from build123d import *

# Parameters (mm, degrees)
SKETCH2_R           = 41.275
SKETCH2_R_2         = 38.1
SKETCH2_R_3         = 34.925
BOSS_EXTRUDE1_DEPTH = 3.175
SKETCH3_R           = 1.5875
BOSS_EXTRUDE2_DEPTH = 3.175
CUT_EXTRUDE1_DEPTH  = 3.175


with BuildPart() as part:
    # Sketch2 → Boss-Extrude1 (new body)
    with BuildSketch(Plane.XY):
        Circle(SKETCH2_R)
        Circle(SKETCH2_R_2, mode=Mode.SUBTRACT)
        Circle(SKETCH2_R_2)
        Circle(SKETCH2_R_3, mode=Mode.SUBTRACT)
    extrude(amount=BOSS_EXTRUDE1_DEPTH)

    # Sketch3 → Boss-Extrude2 (add)
    with BuildSketch(Plane.XY.offset(3.175)):
        with BuildLine():
            ThreePointArc((-25.891068033, 32.144645295), (-23.333836091, 34.046405365), (-20.6375, 35.745198541))
            Line((-20.6375, 35.745198541), (-26.9875, 46.743721169))
            Line((-26.9875, 46.743721169), (-32.486761314, 43.568721169))
            Line((-32.486761314, 43.568721169), (-26.136761314, 32.570198541))
            Line((-26.136761314, 32.570198541), (-25.891068033, 32.144645295))
        make_face()
        with Locations((-28.149630657, 42.406590512)):
            Circle(SKETCH3_R, mode=Mode.SUBTRACT)
        with BuildLine():
            Line((26.9875, 46.743721169), (20.6375, 35.745198541))
            ThreePointArc((20.6375, 35.745198541), (23.333836091, 34.046405365), (25.891068033, 32.144645295))
            Line((25.891068033, 32.144645295), (26.136761314, 32.570198541))
            Line((26.136761314, 32.570198541), (32.486761314, 43.568721169))
            Line((32.486761314, 43.568721169), (26.9875, 46.743721169))
        make_face()
        with Locations((28.149630657, 42.406590512)):
            Circle(SKETCH3_R, mode=Mode.SUBTRACT)
    extrude(amount=-BOSS_EXTRUDE2_DEPTH)

    # Sketch5 → Cut-Extrude1 (cut)
    with BuildSketch(Plane.XY.offset(3.175)):
        with BuildLine():
            Line((-20.6375, 35.745198541), (0, 0))
            Line((0, 0), (20.6375, 35.745198541))
            ThreePointArc((20.6375, 35.745198541), (0, 41.275), (-20.6375, 35.745198541))
        make_face()
    extrude(amount=-CUT_EXTRUDE1_DEPTH, mode=Mode.SUBTRACT)


solid = part.part
Verification items for the finished model (mm, model axes). A direction names the side the tool comes from. Coordinates: 2 decimals unless noted, no trailing zeros. Write each loop counter-clockwise with the first axis right and the second up, starting at its lowest first coordinate (ties: lowest second). Pieces come first, ordered by that corner, then holes. Notation, with made-up numbers: M 56.25,85.25 L 103.25,85.25 A31 ccw 103.25,113.25 Z; hole C -21,47.25 d4. An arc over 180 degrees is marked long. Use a Markdown table: item, result.
Q1. Sectioned sample at C-C, the plane y = 22. Record the boundary of the cut face in (x, z) (3 decimals).
Reply:
| item | result |
|---|---|
| outline | M -34.923,0 L -27.125,0 L -27.125,3.175 L -34.923,3.175 Z; M 27.125,0 L 34.923,0 L 34.923,3.175 L 27.125,3.175 Z |
Q2. Sectioned sample at D-D, the plane x = 0. Record the boundary of the cut face in (y, z) (3 decimals).
Reply:
| item | result |
|---|---|
| outline | M -41.275,0 L -34.925,0 L -34.925,3.175 L -41.275,3.175 Z |
Q3. Sectioned sample at A-A, the plane y = 0. Record the boundary of the cut face in (x, z) (3 decimals), plus the area to 3 significant figures.
Reply:
| item | result |
|---|---|
| outline | M -41.275,0 L -34.925,0 L -34.925,3.175 L -41.275,3.175 Z; M 34.925,0 L 41.275,0 L 41.275,3.175 L 34.925,3.175 Z |
| area | 40.3 mm² |
Q4. Go/stop test with flat-tipped pins: P1, Ø1.5, axis at x = -2.5, z = 1, coming from the -Y side; P2, Ø1, axis at y = 13, z = 2, coming from the -X side; P3, Ø1, axis at x = 32.5, z = 2.5, coming from the +Y side. Record where each tip stops, or that it passes through.
Reply:
| item | result |
|---|---|
| P1 | stops at y = -41.24 |
| P2 | stops at x = -39.34 |
| P3 | stops at y = 43.85 |
Q5. Draft check along X on faces 1 (the face through (-19, -30, 0)), 2 (the face through (29.78, 45.13, 1.61)), 3 (the face through (28.882, 40.998, 1.61)). Enter one of: +X half, -X half, draft (parallel to the pull), parting line (faces both ways), or undercut.
Reply:
| item | result |
|---|---|
| face 1 | draft |
| face 2 | +X half |
| face 3 | undercut |
Q6. Sectioned sample at B-B, the plane z = 2.35. Count the separate pieces of the cut face and the enclosed holes in it, plus the area to 3 significant figures.
Reply:
| item | result |
|---|---|
| separate pieces | 1 |
| enclosed holes | 2 |
| area | 1,410 mm² |
Q7. Thickness scan on line 1 (Y direction, x = -27, z = 2.55); line 2 (X direction, y = 0, z = 1) (3 decimals); line 3 (Y direction, x = 30, z = 2.85). Record the ranges inside material, lowest first.
Reply:
| item | result |
|---|---|
| line 1 | y = -31.22 to -22.15, 22.15 to 31.22, 34.07 to 41.31, 43.5 to 46.74 |
| line 2 | x = -41.275 to -34.925, 34.925 to 41.275 |
| line 3 | y = -28.35 to -17.88, 17.88 to 28.35, 39.26 to 45 |
Q8. Set-up check for faces 4 (the face through (22.16, 38.38, 1.61)), 5 (the face through (-1.3, -34.9, 1.6)): record each of +Z, -Z, +X, -X, +Y, -Y from which the full face is reachable in a straight line by a thin tool's end or side.
Reply:
| item | result |
|---|---|
| face 4 | +Z, -Z, +Y |
| face 5 | +Z, -Z |
